Study the drawing (mm; zero at the part's minimum x, y, z) and answer. A direction names the side the tool comes from. Give positions to 0.01 mm unless a question says otherwise; leave off trailing zeros. Write each loop counter-clockwise with the first axis right and the second up, starting at its lowest first coordinate (ties: lowest second). Pieces come first, ordered by that corner, then holes. Notation, with made-up numbers: (50.25, -17.75) - (91.25, -17.75) arc R19 cw to (91.25, -3.75) - close; hole circle Ø6 at (25, 86.5). An arc over 180 degrees is marked (long way). One line per item, written item: value. Start each with the question number.
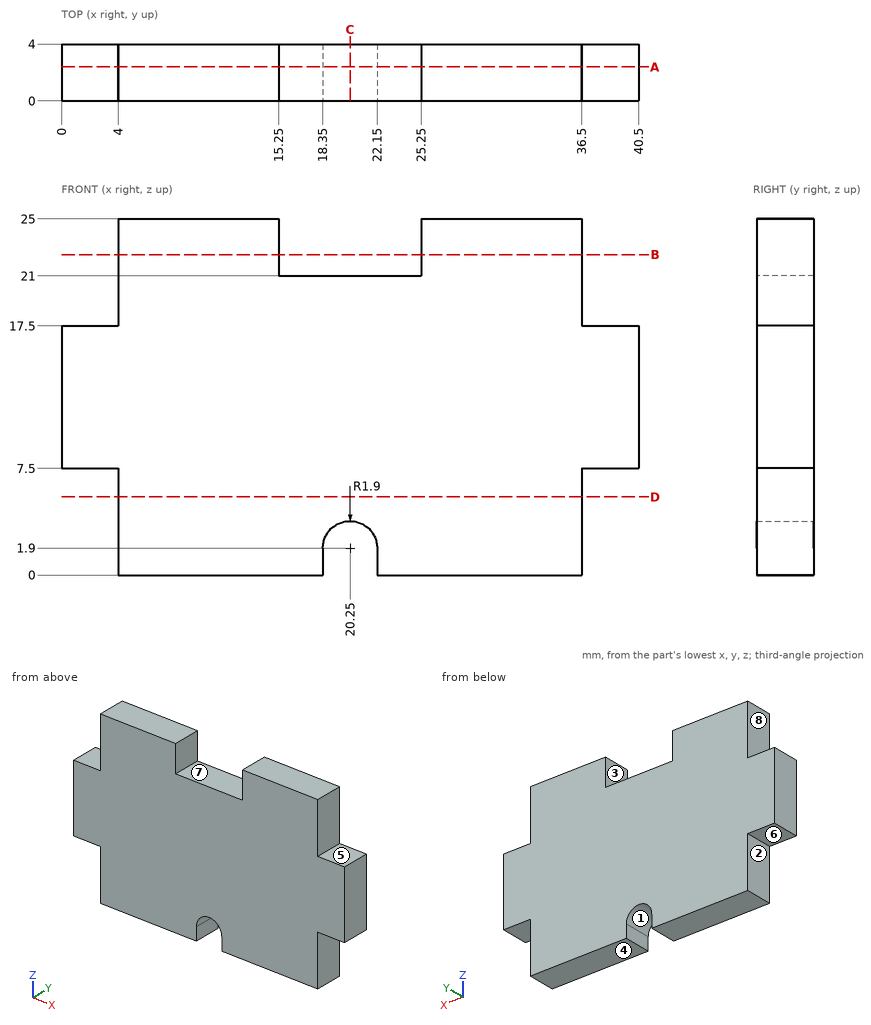
Item 1: Find section B-B on z = 22.5. Determine the outline of the cut face in (x, y).
Item 2: The mould has two halves that part along X. Classify the marked faces 1, 2, 3 and 4: +X half, -X half, draft (parallel to the pull), parting line (faces both ways), or undercut.
Item 3: Find section A-A on y = 2.4. Determine the outline of the cut face in (x, z), plus the area to 3 significant figures.
Item 4: Each of these flat-tipped pins is pushed along its axis until it touches: pin 1 Ø1.5 at (x, y) = (17, 1.5) entering from +Z; pin 2 Ø2 at (y, z) = (1, 23.5) entering from +X; pin 3 Ø1 at (y, z) = (1.5, 1) entering from -X. Where does it stop, or does it pass through?
Item 5: For the marked faces 5, 6, 7 and 8, determine the directions among +Z, -Z, +X, -X, +Y, -Y from which every point of the face is accessible in a straight line to the end or side of a thin tool.
Item 6: Find section C-C on x = 20.25. Determine the outline of the cut face in (y, z), plus the area to 3 significant figures.
Item 7: Straight lines are drawn through the part: line 1 along X through (y, z) = (2.65, 24); line 2 along X through (y, z) = (2.85, 18.75); line 3 along Z through (x, y) = (38, 0.6). For each, find the intervals that lie inside material, in ascending order.
Item 8: Find section D-D on z = 5.5. Determine the outline of the cut face in (x, y), plus the area to 3 significant figures.
Values:
1. outline: (4, 0) - (15.25, 0) - (15.25, 4) - (4, 4) - close; (25.25, 0) - (36.5, 0) - (36.5, 4) - (25.25, 4) - close
2. face 1: undercut
2. face 2: -X half
2. face 3: undercut
2. face 4: draft
3. outline: (0, 7.5) - (4, 7.5) - (4, 0) - (18.35, 0) - (18.35, 1.9) arc R1.9 cw to (22.15, 1.9) - (22.15, 0) - (36.5, 0) - (36.5, 7.5) - (40.5, 7.5) - (40.5, 17.5) - (36.5, 17.5) - (36.5, 25) - (25.25, 25) - (25.25, 21) - (15.25, 21) - (15.25, 25) - (4, 25) - (4, 17.5) - (0, 17.5) - close
3. area: 840 mm^2
4. pin 1: z = 21
4. pin 2: x = 36.5
4. pin 3: x = 4
5. face 5: +Z, +X, +Y, -Y
5. face 6: -Z, -X, +Y, -Y
5. face 7: +Z, +Y, -Y
5. face 8: +Z, -X, +Y, -Y
6. outline: (0, 3.8) - (4, 3.8) - (4, 21) - (0, 21) - close
6. area: 68.8 mm^2
7. line 1: 4 to 15.25, 25.25 to 36.5
7. line 2: 4 to 36.5
7. line 3: 7.5 to 17.5
8. outline: (4, 0) - (36.5, 0) - (36.5, 4) - (4, 4) - close
8. area: 130 mm^2
